The drawing under review shows one solid part. Ordinate dimensions are in mm from its lowest x, y, z. A direction names the side the tool comes from. Coordinates: 2 decimals unless noted, no trailing zeros. Order: outer loops, then holes, each group sorted by start corner. A loop starts at its lowest first (then second) coordinate and runs counter-clockwise, first axis right, second up. Notation, with made-up numbers: M -4.75,69 L 52.25,69 A30 cw 52.25,94 Z; hole C 20.5,5.25 d5. An arc over 180 degrees is marked long. Answer as a JSON object with one key per item and string values.
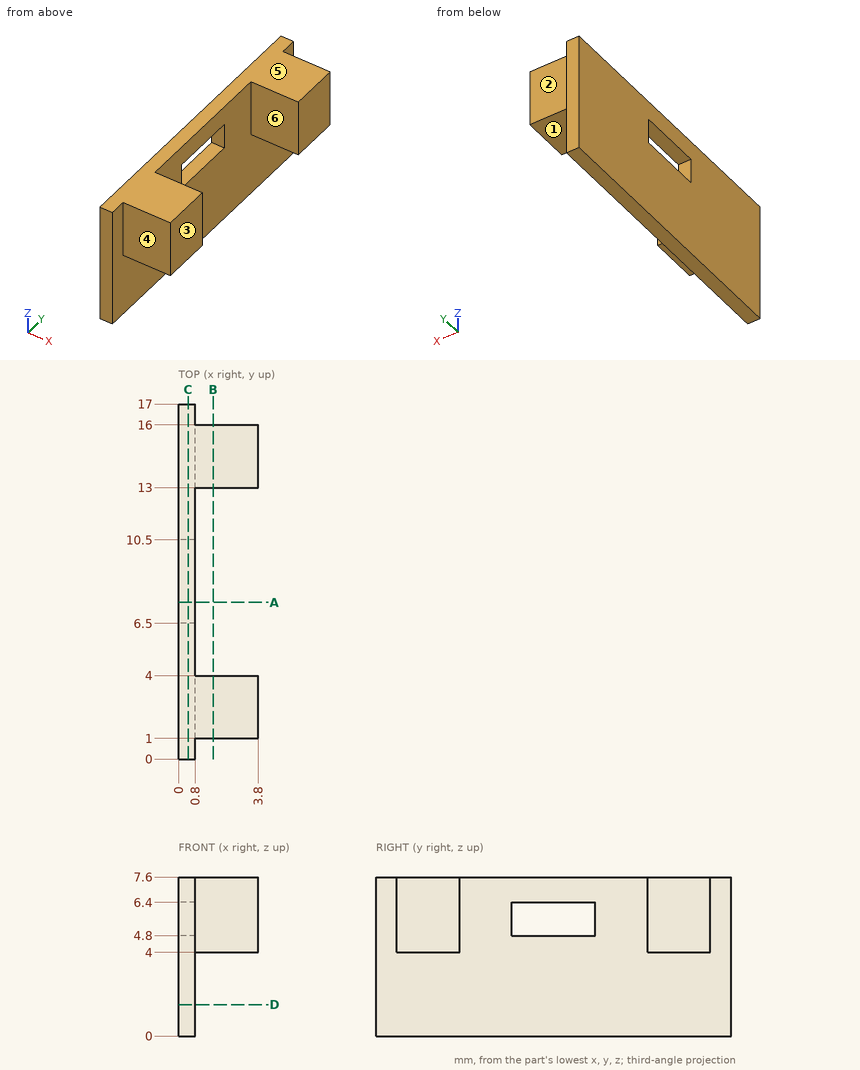
1) Add section B-B (x = 1.65). State the section outline as (y, z) points, and give its area (3 significant figures).
Taken from the geometry:
{"outline": "M 1,4 L 4,4 L 4,7.6 L 1,7.6 Z; M 13,4 L 16,4 L 16,7.6 L 13,7.6 Z", "area": "21.6 mm2"}
2) Insertion check: pin 1 Ø2.5 at (y, z) = (10.5, 4.5) entering from +X; pin 2 Ø0.9 at (x, z) = (2.5, 5) entering from -Y; pin 3 Ø0.9 at (x, y) = (3, 2) entering from -Z; pin 4 Ø0.9 at (x, y) = (0.5, 9) entering from -Z. Each pin has a flat end and moves straight along its axis. Give the tip position at first contact, or say it passes through.
Taken from the geometry:
{"pin 1": "stops at x = 0.8", "pin 2": "stops at y = 1", "pin 3": "stops at z = 4", "pin 4": "stops at z = 0"}
3) Add section D-D (z = 1.5). State the section outline as (x, y) points.
Taken from the geometry:
{"outline": "M 0,0 L 0.8,0 L 0.8,17 L 0,17 Z"}
4) Mouldability with a two-part tool opening along Y and no side actions: class the marked faces 4, 5 and 6 as released by +Y, released by -Y, zero draft, split by the parting line, or undercut.
Taken from the geometry:
{"face 4": "released by -Y", "face 5": "zero draft", "face 6": "undercut"}
5) To check wall thickness, follow L1, parallel to Y at x = 1.65, z = 4.5; L2, parallel to Y at x = 0.5, z = 5.5; L3, parallel to X at y = 9.5, z = 7. State the ranges of each line that lie inside material, in increasing order.
Taken from the geometry:
{"L1": "y = 1 to 4, 13 to 16", "L2": "y = 0 to 6.5, 10.5 to 17", "L3": "x = 0 to 0.8"}
6) Add section A-A (y = 7.5). State the section outline as (x, z) points.
Taken from the geometry:
{"outline": "M 0,0 L 0.8,0 L 0.8,4.8 L 0,4.8 Z; M 0,6.4 L 0.8,6.4 L 0.8,7.6 L 0,7.6 Z"}
7) Tool access review of the marked faces 1, 2 and 3: name each direction out of +Z, -Z, +X, -X, +Y, -Y from which nothing blocks a thin tool from reaching the whole face with its end or side.
Taken from the geometry:
{"face 1": "-Z, +X, +Y, -Y", "face 2": "+Z, -Z, +X, +Y", "face 3": "+Z, -Z, +X, +Y, -Y"}
8) Add section C-C (x = 0.45). State the section outline as (y, z) points.
Taken from the geometry:
{"outline": "M 0,0 L 17,0 L 17,7.6 L 0,7.6 Z; hole M 6.5,4.8 L 10.5,4.8 L 10.5,6.4 L 6.5,6.4 Z"}
